Model file for the job. Use its own axes, mm. Face numbers are marked on the shaded views. Round coordinates to 2 decimals unless told otherwise and drop trailing zeros. Loops run counter-clockwise (first coordinate to the right, second up) from the corner with the lowest first, then second, coordinate; pieces in that order, holes last. Notation, with made-up numbers: M 83,10 L 101,10 A19 cw 101,43 Z; hole C 50,-12.5 d10. An arc over 180 degrees is marked long. Use a Markdown table: item, result. Add a question column.
Item 1: Wall check: L1, parallel to Y at x = 0, z = -9.5; L2, parallel to Y at x = 2, z = 4.5; L3, parallel to Z at x = 0, y = -21. Give the ranges that are in metal, low to high. Write a range as from..to.
Item 2: Two-plate mould, pull along Y, no slides. Class the marked faces 1, 2, 3 and 4: +Y half, -Y half, draft (parallel to the pull), parting line (faces both ways), or undercut.
Item 3: Saw through at D-D on z = -6.5. Write the cut outline in (x, y), then the cut area to 3 significant figures.
Item 4: Saw through at A-A on z = 3.25. Give the number of separate pieces and of enclosed holes in the cut face, then the cut area to 3 significant figures.
Item 5: Saw through at C-C on x = -14. Write the cut outline in (y, z), then the cut area to 3 significant figures.
Item 6: Saw through at B-B on y = -13.5. Write the cut outline in (x, z).
Item 7: Pin check, flat tips, straight feed: P1, Ø3, axis at x = 20.5, y = 12.5, coming from the -Z side; P2, Ø4, axis at y = 7.5, z = 2.5, coming from the -X side; P3, Ø6, axis at x = -2, y = -19.5, coming from the +Z side. Stop position of each tip, or through.
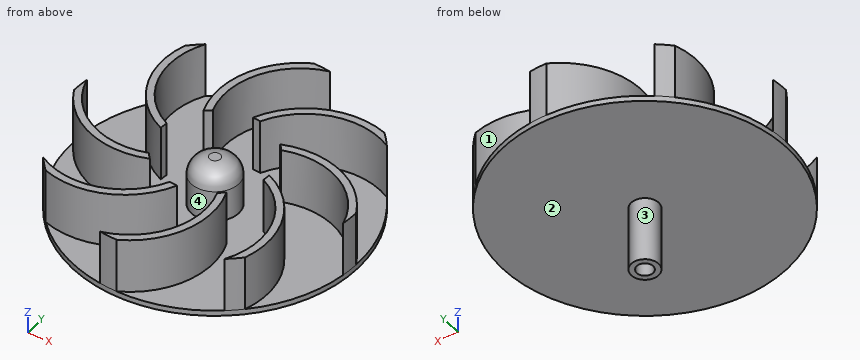
```python
from build123d import *

# Parameters (mm, degrees)
BOSS_EXTRUDE1_DEPTH = 10
CIRPATTERN1_COUNT   = 8
SKETCH4_R           = 2.5
BOSS_EXTRUDE2_DEPTH = 11.83333333
SKETCH5_R           = 1.5
CUT_EXTRUDE1_DEPTH  = 10


with BuildPart() as part:
    # Sketch1 → Revolve2 (revolve)
    with BuildSketch(Plane(origin=(0, 0, 0), x_dir=(0, 0, -1), z_dir=(1, 0, 0))):
        with BuildLine():
            Line((0, 0), (0, 26))
            Line((0, 26), (-1, 26))
            Line((-1, 26), (-1, 4.333333333))
            Line((-1, 4.333333333), (-6.666666667, 4.333333333))
            ThreePointArc((-6.666666667, 4.333333333), (-9.023689271, 3.357022604), (-10, 1))
            Line((-10, 1), (-10, 0))
            Line((-10, 0), (0, 0))
        make_face()
    revolve(axis=Axis((0, 0, 10), (0, 0, -1)))

    # Sketch3 → Boss-Extrude1 (add)
    with BuildSketch(Plane.XY.offset(1)):
        with BuildLine():
            ThreePointArc((-5.998935548, 8.000798228), (-6.551514834, 7.554975406), (-7.071067812, 7.071067812))
            ThreePointArc((-7.071067812, 7.071067812), (-7.201026268, 17.904810567), (0, 26))
            ThreePointArc((0, 26), (1.573713281, 25.952329886), (3.141655863, 25.809494347))
            ThreePointArc((3.141655863, 25.809494347), (-5.308082056, 18.896330591), (-5.998935548, 8.000798228))
        make_face()
    boss_extrude1 = extrude(amount=BOSS_EXTRUDE1_DEPTH)

    # CirPattern1: Boss-Extrude1 ×8 about axis
    cirpattern1_axis = Axis((0, 0, 0), (0, 0, 1))
    for i in range(1, CIRPATTERN1_COUNT):
        add(boss_extrude1.rotate(cirpattern1_axis, i * 360 / CIRPATTERN1_COUNT))

    # Sketch4 → Boss-Extrude2 (add)
    with BuildSketch(Plane(origin=(0, 0, 0), x_dir=(-1, 0, 0), z_dir=(0, 0, -1))):
        Circle(SKETCH4_R)
    extrude(amount=BOSS_EXTRUDE2_DEPTH)

    # Sketch5 → Cut-Extrude1 (cut)
    with BuildSketch(Plane(origin=(0, 0, -11.83333333), x_dir=(-1, 0, 0), z_dir=(0, 0, -1))):
        Circle(SKETCH5_R)
    extrude(amount=-CUT_EXTRUDE1_DEPTH, mode=Mode.SUBTRACT)


solid = part.part
```
Entries:
| question | item | result |
|---|---|---|
| 1 | L1 | -2.5..-1.5, 1.5..2.5 |
| 1 | L2 | -24.77..-23.07, -3.84..3.84, 11.01..13.37, 25.43..25.92 |
| 1 | L3 | 0..1 |
| 2 | face 1 | undercut |
| 2 | face 2 | draft |
| 2 | face 3 | parting line |
| 2 | face 4 | undercut |
| 3 | outline | C 0,0 d5; hole C 0,0 d3 |
| 3 | area | 12.6 mm2 |
| 4 | separate pieces | 9 |
| 4 | enclosed holes | 0 |
| 4 | area | 297 mm2 |
| 5 | outline | M -21.91,0 L 21.91,0 L 21.91,1 L 4.37,1 L 4.37,11 L 2.52,11 L 2.52,1 L -6.75,1 L -6.75,11 L -8.09,11 L -8.09,1 L -17.77,1 L -17.77,11 L -19.1,11 L -19.1,1 L -21.91,1 Z |
| 5 | area | 89.0 mm2 |
| 6 | outline | M -22.22,0 L 22.22,0 L 22.22,1 L 19.1,1 L 19.1,11 L 17.77,11 L 17.77,1 L 8.13,1 L 8.13,11 L 6.79,11 L 6.79,1 L -2.1,1 L -2.1,11 L -3.87,11 L -3.87,1 L -22.22,1 Z |
| 7 | P1 | z = 0 |
| 7 | P2 | x = -25.26 |
| 7 | P3 | z = 1 |
